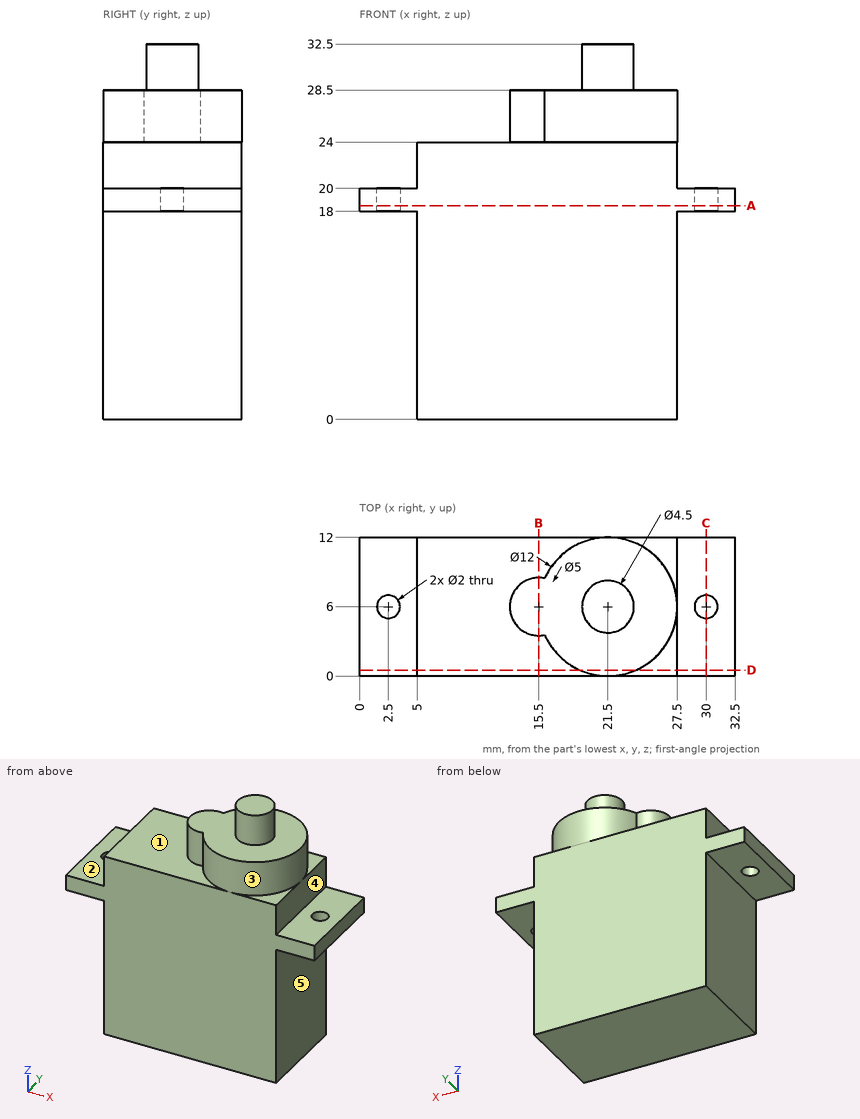
Input: dimensioned drawing with shaded views. Units: mm. Origin: part minimum x, y, z. A direction names the side the tool comes from. Round coordinates to 2 decimals unless told otherwise and drop trailing zeros. Loops run counter-clockwise (first coordinate to the right, second up) from the corner with the lowest first, then second, coordinate; pieces in that order, holes last. Notation, with made-up numbers: (71, 46) -> (124, 46) arc R22 ccw to (124, 60) -> close; hole circle Ø1 at (-27, -27.75). An arc over 180 degrees is marked (long way). Answer as a JSON object with one key per item and string values. Group by question number.
Q1. Access query for the marked faces 1, 2, 3, 4 and 5. Directions: +Z, -Z, +X, -X, +Y, -Y. A direction counts if a zero-diameter tool reaches every point of the face in a straight line with its end or side. Return the directions, or none.
Q2. Section query A-A (z = 18.5). Output: boundary loops of the cut face in (x, y), plus the area to 3 significant figures.
Q3. Section query D-D (y = 0.5). Output: boundary loops of the cut face in (x, z).
Q4. Section query C-C (x = 30). Output: boundary loops of the cut face in (y, z).
Q5. Ray query, line 1 (Y direction, x = 2.5, z = 19.35); line 2 (Z direction, x = 11, y = 9); line 3 (Z direction, x = 22.5, y = 8.5). Return the intervals inside material, ascending. Write a range as from..to.
Q6. Contact query for flat-ended pins moving along their axis: P1, Ø2.5, axis at x = 2.5, y = 6, coming from the +Z side; P2, Ø1.5, axis at y = 8.5, z = 12, coming from the -X side; P3, Ø6, axis at x = 14.5, y = 3.5, coming from the +Z side. Output: stop coordinate, or through.
Q7. Section query B-B (x = 15.5). Output: boundary loops of the cut face in (y, z).
Completed:
{
 "1": {"face 1": "+Z, -X", "face 2": "+Z, -X, +Y, -Y", "face 3": "+Z", "face 4": "+Z, +X, +Y, -Y", "face 5": "-Z, +X, +Y, -Y"},
 "2": {"outline": "(0, 0) -> (32.5, 0) -> (32.5, 12) -> (0, 12) -> close; hole circle Ø2 at (2.5, 6); hole circle Ø2 at (30, 6)", "area": "384 mm²"},
 "3": {"outline": "(0, 18) -> (5, 18) -> (5, 0) -> (27.5, 0) -> (27.5, 18) -> (32.5, 18) -> (32.5, 20) -> (27.5, 20) -> (27.5, 24) -> (23.9, 24) -> (23.9, 28.5) -> (19.1, 28.5) -> (19.1, 24) -> (5, 24) -> (5, 20) -> (0, 20) -> close"},
 "4": {"outline": "(0, 18) -> (5, 18) -> (5, 20) -> (0, 20) -> close; (7, 18) -> (12, 18) -> (12, 20) -> (7, 20) -> close"},
 "5": {"line 1": "0..5, 7..12", "line 2": "0..24", "line 3": "0..28.5"},
 "6": {"P1": "z = 20", "P2": "x = 5", "P3": "z = 28.5"},
 "7": {"outline": "(0, 0) -> (12, 0) -> (12, 24) -> (8.5, 24) -> (8.5, 28.5) -> (3.5, 28.5) -> (3.5, 24) -> (0, 24) -> close"}
}
